Verification items for the finished model (mm, model axes). Give positions to 0.01 mm unless a question says otherwise; leave off trailing zeros. Order: outer loops, then holes, each group sorted by start corner. A loop starts at its lowest first (then second) coordinate and runs counter-clockwise, first axis right, second up. Notation, with made-up numbers: M 76.25,15 L 125.25,15 A21 cw 125.25,22 Z; hole C -20.75,59 d9. An arc over 180 degrees is marked long. Answer as a JSON object with one key per item and string values.
```python
from build123d import *

# Parameters (mm, degrees)
EXTRUDE_1_DEPTH             = 2.54
SKETCH_2_W                  = 0.599854391
SKETCH_2_H                  = 0.599854392
EXTRUDE_2_DEPTH             = 5.08
SKETCH_4_W                  = 0.2
SKETCH_4_H                  = 5
CUT_EXTRUDE_2_DEPTH         = 0.2
CUT_EXTRUDE_3_REACH         = 9.607
SKETCH_5_W                  = 0.2
SKETCH_5_H                  = 0.2
PATTERN_LINEAR_2_COUNT      = 3
PATTERN_LINEAR_2_PITCH      = 2.54
CHAMFER_1_SIZE              = 0.2
CHAMFER_2_SIZE              = 0.2
PATTERN_LINEAR_3_COUNT      = 4
PATTERN_LINEAR_3_PITCH      = 2.54
PATTERN_LINEAR_3_COUNT_DIR2 = 2
PATTERN_LINEAR_3_PITCH_DIR2 = 2.54
FILLET_4_R                  = 0.05
SKETCH_6_W                  = 13.31877373
SKETCH_6_H                  = 4.876948745
CUT_EXTRUDE_4_DEPTH         = 10


with BuildPart() as part:
    # Sketch 1 → Extrude 1 (new body)
    with BuildSketch(Plane.XY):
        Polygon((5.08, 2.5), (-5.08, 2.5), (-5.08, 0), (-5.08, -2.5), (5.08, -2.5), (5.08, 0), align=None)
    extrude(amount=EXTRUDE_1_DEPTH)

    # Sketch 2 → Extrude 2 (add, symmetric)
    with BuildSketch(Plane.XY.offset(2.54)):
        with Locations((-3.805698419, 1.27)):
            Rectangle(SKETCH_2_W, SKETCH_2_H)
    extrude_2 = extrude(amount=EXTRUDE_2_DEPTH, both=True)

    # Sketch 4 → Cut-Extrude 2 (cut)
    with BuildSketch(Plane.XY.offset(2.54)):
        with Locations((-2.54, 0)):
            Rectangle(SKETCH_4_W, SKETCH_4_H)
    cut_extrude_2 = extrude(amount=-CUT_EXTRUDE_2_DEPTH, mode=Mode.SUBTRACT)

    # Sketch 5 → Cut-Extrude 3 (cut, up to next)
    with BuildSketch(Plane.XY.offset(2.54), mode=Mode.PRIVATE) as cut_extrude_3_sk1:
        with Locations((-2.54, 2.4)):
            Rectangle(SKETCH_5_W, SKETCH_5_H)
    cut_extrude_3_tool1 = extrude(cut_extrude_3_sk1.sketch, amount=-CUT_EXTRUDE_3_REACH, mode=Mode.PRIVATE) & part.part
    # Sketch 5 → Cut-Extrude 3 (cut, up to next)
    with BuildSketch(Plane.XY.offset(2.54), mode=Mode.PRIVATE) as cut_extrude_3_sk2:
        with Locations((-2.54, -2.4)):
            Rectangle(SKETCH_5_W, SKETCH_5_H)
    cut_extrude_3_tool2 = extrude(cut_extrude_3_sk2.sketch, amount=-CUT_EXTRUDE_3_REACH, mode=Mode.PRIVATE) & part.part
    cut_extrude_3_1 = cut_extrude_3_tool1.solids().sort_by_distance((-2.54, 2.4, 2.54))[0]
    add(cut_extrude_3_1, mode=Mode.SUBTRACT)
    cut_extrude_3_2 = cut_extrude_3_tool2.solids().sort_by_distance((-2.54, -2.4, 2.54))[0]
    add(cut_extrude_3_2, mode=Mode.SUBTRACT)
    cut_extrude_3 = cut_extrude_3_1 + cut_extrude_3_2  # Cut-Extrude 3 as one shape, for the pattern or mirror that repeats it

    # Pattern Linear 2: Cut-Extrude 2, Cut-Extrude 3 ×3
    with Locations(*[(i * PATTERN_LINEAR_2_PITCH, 0, 0) for i in range(1, PATTERN_LINEAR_2_COUNT)]):
        add(cut_extrude_2, mode=Mode.SUBTRACT)
        add(cut_extrude_3, mode=Mode.SUBTRACT)

    # Chamfer 1
    chamfer_1_edges = [part.edges().sort_by_distance(p)[0] for p in [
        (5.08, -1.25, 2.54),
        (-5.08, 2.5, 1.27),
        (5.08, 2.5, 1.27),
        (5.08, -2.5, 1.27),
        (-5.08, -2.5, 1.27),
        (-5.08, -1.25, 2.54),
    ]]
    chamfer(chamfer_1_edges, length=CHAMFER_1_SIZE)

    # Chamfer 2
    chamfer_2_edges = [part.edges().sort_by_distance(p)[0] for p in [
        (-2.64, -2.5, 1.27),
        (2.44, -2.5, 1.27),
        (0.1, -2.5, 1.27),
        (2.64, -2.5, 1.27),
        (-0.1, -2.5, 1.27),
        (-2.44, -2.5, 1.27),
        (2.64, 0, 2.54),
        (-2.64, 0, 2.54),
        (-0.1, 0, 2.54),
        (-2.44, 0, 2.54),
        (2.44, 0, 2.54),
        (0.1, 0, 2.54),
        (2.64, 2.5, 1.27),
        (-0.1, 2.5, 1.27),
        (-2.44, 2.5, 1.27),
        (2.44, 2.5, 1.27),
        (0.1, 2.5, 1.27),
        (-2.64, 2.5, 1.27),
    ]]
    chamfer(chamfer_2_edges, length=CHAMFER_2_SIZE - 0.0001)  # a hair under: the kernel refuses the full size

    # Pattern Linear 3: Extrude 2 4 × 2
    with Locations(*[(i * PATTERN_LINEAR_3_PITCH, -j * PATTERN_LINEAR_3_PITCH_DIR2, 0) for i in range(PATTERN_LINEAR_3_COUNT) for j in range(PATTERN_LINEAR_3_COUNT_DIR2) if (i, j) != (0, 0)]):
        add(extrude_2)

    # Fillet 4
    fillet_4_edges = [part.edges().sort_by_distance(p)[0] for p in [
        (-3.805698419, -0.970072804, -2.54),
        (-4.105625614, -1.27, -2.54),
        (-3.805698419, -1.569927196, -2.54),
        (-3.505771223, -1.27, -2.54),
        (-3.805698419, -0.970072804, 7.62),
        (-4.105625614, -1.27, 7.62),
        (-3.805698419, -1.569927196, 7.62),
        (-3.505771223, -1.27, 7.62),
        (-1.265698419, 1.569927196, -2.54),
        (-1.565625614, 1.27, -2.54),
        (-1.265698419, 0.970072804, -2.54),
        (-0.965771223, 1.27, -2.54),
        (-1.265698419, 1.569927196, 7.62),
        (-1.565625614, 1.27, 7.62),
        (-1.265698419, 0.970072804, 7.62),
        (-0.965771223, 1.27, 7.62),
        (-1.265698419, -0.970072804, -2.54),
        (-1.565625614, -1.27, -2.54),
        (-1.265698419, -1.569927196, -2.54),
        (-0.965771223, -1.27, -2.54),
        (-1.265698419, -0.970072804, 7.62),
        (-1.565625614, -1.27, 7.62),
        (-1.265698419, -1.569927196, 7.62),
        (-0.965771223, -1.27, 7.62),
        (1.274301581, 1.569927196, -2.54),
        (0.974374386, 1.27, -2.54),
        (1.274301581, 0.970072804, -2.54),
        (1.574228777, 1.27, -2.54),
        (1.274301581, 1.569927196, 7.62),
        (0.974374386, 1.27, 7.62),
        (1.274301581, 0.970072804, 7.62),
        (1.574228777, 1.27, 7.62),
        (1.274301581, -0.970072804, -2.54),
        (0.974374386, -1.27, -2.54),
        (1.274301581, -1.569927196, -2.54),
        (1.574228777, -1.27, -2.54),
        (1.274301581, -0.970072804, 7.62),
        (0.974374386, -1.27, 7.62),
        (1.274301581, -1.569927196, 7.62),
        (1.574228777, -1.27, 7.62),
        (3.814301581, 1.569927196, -2.54),
        (3.514374386, 1.27, -2.54),
        (3.814301581, 0.970072804, -2.54),
        (4.114228777, 1.27, -2.54),
        (3.814301581, 1.569927196, 7.62),
        (3.514374386, 1.27, 7.62),
        (3.814301581, 0.970072804, 7.62),
        (4.114228777, 1.27, 7.62),
        (3.814301581, -0.970072804, -2.54),
        (3.514374386, -1.27, -2.54),
        (3.814301581, -1.569927196, -2.54),
        (4.114228777, -1.27, -2.54),
        (3.814301581, -0.970072804, 7.62),
        (3.514374386, -1.27, 7.62),
        (3.814301581, -1.569927196, 7.62),
        (4.114228777, -1.27, 7.62),
    ]]
    fillet(fillet_4_edges, radius=FILLET_4_R)

    # Sketch 6 → Cut-Extrude 4 (cut)
    with BuildSketch(Plane.XZ.offset(2.5)):
        with Locations((0.654637262, -4.038474373)):
            Rectangle(SKETCH_6_W, SKETCH_6_H)
    extrude(amount=-CUT_EXTRUDE_4_DEPTH, mode=Mode.SUBTRACT)


solid = part.part
```
Q1. Material ranges on L1, parallel to X at y = 1.25, z = 2.75; L2, parallel to Z at x = -1.5, y = 0.4; L3, parallel to Z at x = 2.5, y = 0.85, recorded low to high.
Resolved:
{"L1": "x = -4.11 to -3.51, -1.57 to -0.97, 0.97 to 1.57, 3.51 to 4.11", "L2": "z = 0 to 2.54", "L3": "z = 0 to 2.34"}
Q2. Gauge pin test, flat ends, axial feed: pin 1 Ø1 at (x, y) = (-3.5, 2) entering from +Z; pin 2 Ø0.7 at (x, z) = (1, 5.5) entering from +Y; pin 3 Ø0.5 at (x, z) = (-1.5, -1) entering from -Y; pin 4 Ø0.5 at (y, z) = (1.5, -0.5) entering from -X. Record the tip position at first contact, or that the pin passes through.
Resolved:
{"pin 1": "stops at z = 7.62", "pin 2": "stops at y = 1.57", "pin 3": "stops at y = -1.57", "pin 4": "stops at x = -4.11"}
Q3. Section check A-A on z = 3. Count the separate pieces of the cut face and the enclosed holes in it, then the cut area to 3 significant figures.
Resolved:
{"separate pieces": "8", "enclosed holes": "0", "area": "2.88 mm²"}
Q4. Section check B-B on x = 1.25. Record the cut outline in (y, z).
Resolved:
{"outline": "M -2.5,0 L -1.57,0 L -1.57,-1.6 L -0.97,-1.6 L -0.97,0 L 0.97,0 L 0.97,-1.6 L 1.57,-1.6 L 1.57,0 L 2.5,0 L 2.5,2.54 L 1.57,2.54 L 1.57,7.57 A0.05 ccw 1.52,7.62 L 1.02,7.62 A0.05 ccw 0.97,7.57 L 0.97,2.54 L -0.97,2.54 L -0.97,7.57 A0.05 ccw -1.02,7.62 L -1.52,7.62 A0.05 ccw -1.57,7.57 L -1.57,2.54 L -2.5,2.54 Z"}
Q5. Release check for a two-part mould opening along Y. For faces 1 (the face through (5.08, 0, 1)), 2 (the face through (-1, 0, 2.54)), 3 (the face through (-4, 2.5, 1)), 4 (the face through (4, 0, 2.54)) record: +Y half, -Y half, draft (parallel to the pull), parting line (faces both ways), or undercut.
Resolved:
{"face 1": "draft", "face 2": "undercut", "face 3": "+Y half", "face 4": "undercut"}
Q6. Section check D-D on x = -0.75. Record the cut outline in (y, z), then the cut area to 3 significant figures.
Resolved:
{"outline": "M -2.5,0 L 2.5,0 L 2.5,2.54 L -2.5,2.54 Z", "area": "12.7 mm²"}
